Check sheet for the drawn part. Datum: minimum x, y, z corner. Units: mm. A direction names the side the tool comes from. Round coordinates to 2 decimals unless told otherwise and drop trailing zeros. Write each loop counter-clockwise with the first axis right and the second up, starting at its lowest first coordinate (ties: lowest second). Pieces come first, ordered by that corner, then holes.
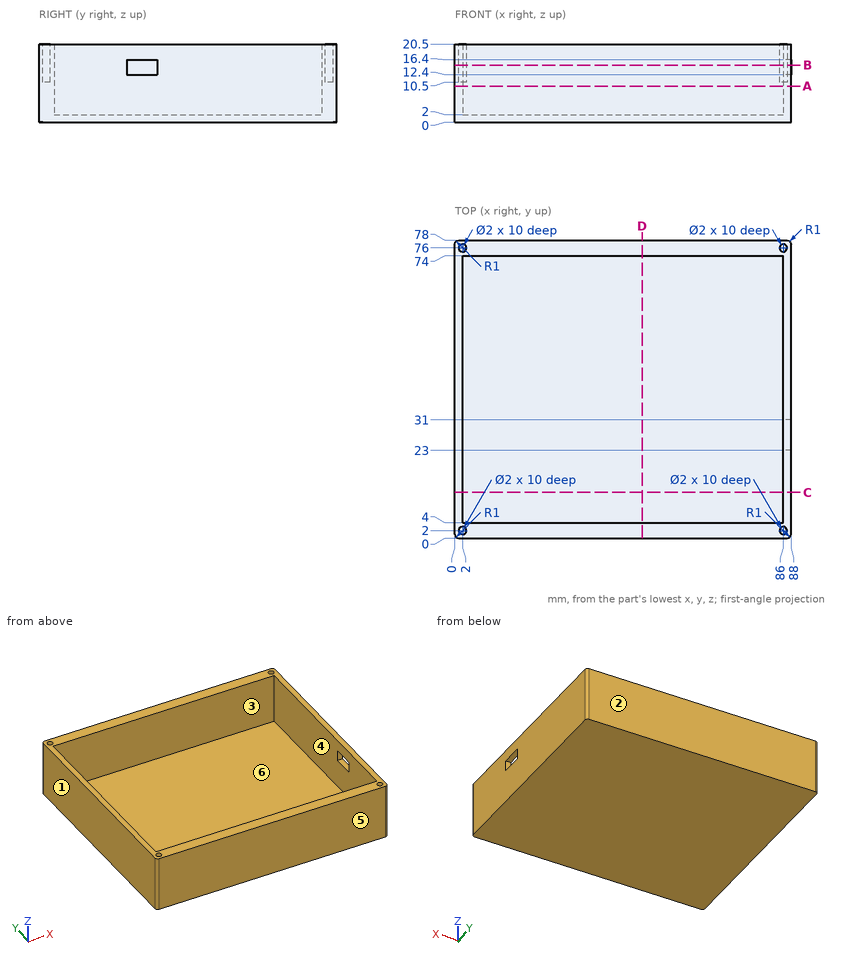
1. Sectioned sample at D-D, the plane x = 49. Enter the section's corners in (y, z), plus the area to 3 significant figures.
2. Release check for a two-part mould opening along X. For the marked faces 1, 2, 3 and 4 record: released by +X, released by -X, zero draft, split by the parting line, or undercut.
3. Sectioned sample at C-C, the plane y = 12. Enter the section's corners in (x, z), plus the area to 3 significant figures.
4. Sectioned sample at B-B, the plane z = 15. Enter the section's corners in (x, y).
5. Sectioned sample at A-A, the plane z = 9.5. Enter the section's corners in (x, y).
6. Set-up check for the marked faces 5 and 6: record each of +Z, -Z, +X, -X, +Y, -Y from which the full face is reachable in a straight line by a thin tool's end or side.
7. Go/stop test with flat-tipped pins: pin 1 (0.6 mm diameter, centred on x = 86, y = 75.5, fed in from +Z); pin 2 (4 mm diameter, centred on x = 53.5, y = 55.5, fed in from +Z). Record where each tip stops, or that it passes through.
8. Scan lines: line 1 along X through (y, z) = (76, 13.25); line 2 along X through (y, z) = (36.5, 15.5); line 3 along Y through (x, z) = (76.5, 4). Record each from-to range of solid material in increasing order.
Computed values:
1. outline: (0, 0) - (78, 0) - (78, 20.5) - (74, 20.5) - (74, 2) - (4, 2) - (4, 20.5) - (0, 20.5) - close
1. area: 304 mm2
2. face 1: released by -X
2. face 2: zero draft
2. face 3: undercut
2. face 4: undercut
3. outline: (0, 0) - (88, 0) - (88, 20.5) - (86, 20.5) - (86, 2) - (2, 2) - (2, 20.5) - (0, 20.5) - close
3. area: 250 mm2
4. outline: (0, 1) arc R1 ccw to (1, 0) - (87, 0) arc R1 ccw to (88, 1) - (88, 23) - (86, 23) - (86, 4) - (2, 4) - (2, 74) - (86, 74) - (86, 31) - (88, 31) - (88, 77) arc R1 ccw to (87, 78) - (1, 78) arc R1 ccw to (0, 77) - close; hole circle Ø2 at (2, 2); hole circle Ø2 at (2, 76); hole circle Ø2 at (86, 2); hole circle Ø2 at (86, 76)
5. outline: (0, 1) arc R1 ccw to (1, 0) - (87, 0) arc R1 ccw to (88, 1) - (88, 77) arc R1 ccw to (87, 78) - (1, 78) arc R1 ccw to (0, 77) - close; hole (2, 4) - (86, 4) - (86, 74) - (2, 74) - close
6. face 5: +Z, -Z, +X, -X, -Y
6. face 6: +Z
7. pin 1: stops at z = 10.5
7. pin 2: stops at z = 2
8. line 1: x = 0 to 1, 3 to 85, 87 to 88
8. line 2: x = 0 to 2, 86 to 88
8. line 3: y = 0 to 4, 74 to 78
